from build123d import *

# Parameters (mm, degrees)
SKETCH1_W           = 200
SKETCH1_H           = 10
BOSS_EXTRUDE1_DEPTH = 66.54
CUT_EXTRUDE1_REACH  = 122.219
SKETCH2_R           = 1.5
LPATTERN1_COUNT     = 4
LPATTERN1_PITCH     = 64
SKETCH3_W           = 200
SKETCH3_H           = 10
CUT_EXTRUDE2_DEPTH  = 3
SKETCH4_W           = 3
SKETCH4_H           = 56.54
BOSS_EXTRUDE2_DEPTH = 8
CUT_EXTRUDE3_REACH  = 213.179
SKETCH5_R           = 1.5


with BuildPart() as part:
    # Sketch1 → Boss-Extrude1 (new body)
    with BuildSketch(Plane(origin=(0, 0, 0), x_dir=(1, 0, 0), z_dir=(0, 1, 0))):
        Rectangle(SKETCH1_W, SKETCH1_H)
    extrude(amount=BOSS_EXTRUDE1_DEPTH)

    # Sketch2 → Cut-Extrude1 (cut, up to next)
    with BuildSketch(Plane(origin=(0, 66.54, 0), x_dir=(1, 0, 0), z_dir=(0, 1, 0)), mode=Mode.PRIVATE) as cut_extrude1_sk1:
        with Locations(Location((-96, 0, 0), (0, 0, 270))):
            Circle(SKETCH2_R)
    cut_extrude1_tool1 = extrude(cut_extrude1_sk1.sketch, amount=-CUT_EXTRUDE1_REACH, mode=Mode.PRIVATE) & part.part
    cut_extrude1 = cut_extrude1_tool1.solids().sort_by_distance((-96, 66.54, 0))[0]
    add(cut_extrude1, mode=Mode.SUBTRACT)

    # LPattern1: Cut-Extrude1 ×4
    with Locations(*[(i * LPATTERN1_PITCH, 0, 0) for i in range(1, LPATTERN1_COUNT)]):
        add(cut_extrude1, mode=Mode.SUBTRACT)

    # Sketch3 → Cut-Extrude2 (cut)
    with BuildSketch(Plane.XY.offset(5)):
        with Locations((0, 5)):
            Rectangle(SKETCH3_W, SKETCH3_H)
    extrude(amount=-CUT_EXTRUDE2_DEPTH, mode=Mode.SUBTRACT)

    # Sketch4 → Boss-Extrude2 (add)
    with BuildSketch(Plane.XY.offset(5)):
        with Locations((-98.5, 38.27)):
            Rectangle(SKETCH4_W, SKETCH4_H)
    extrude(amount=BOSS_EXTRUDE2_DEPTH)

    # Sketch5 → Cut-Extrude3 (cut, up to next)
    with BuildSketch(Plane.ZY.offset(100), mode=Mode.PRIVATE) as cut_extrude3_sk1:
        with Locations((9, 58.27)):
            Circle(SKETCH5_R)
    cut_extrude3_tool1 = extrude(cut_extrude3_sk1.sketch, amount=-CUT_EXTRUDE3_REACH, mode=Mode.PRIVATE) & part.part
    # Sketch5 → Cut-Extrude3 (cut, up to next)
    with BuildSketch(Plane.ZY.offset(100), mode=Mode.PRIVATE) as cut_extrude3_sk2:
        with Locations((9, 13.27)):
            Circle(SKETCH5_R)
    cut_extrude3_tool2 = extrude(cut_extrude3_sk2.sketch, amount=-CUT_EXTRUDE3_REACH, mode=Mode.PRIVATE) & part.part
    add(cut_extrude3_tool1.solids().sort_by_distance((-100, 58.27, 9))[0], mode=Mode.SUBTRACT)
    add(cut_extrude3_tool2.solids().sort_by_distance((-100, 13.27, 9))[0], mode=Mode.SUBTRACT)


solid = part.part
Part model, mm, in its own coordinate system. A direction names the side the tool comes from. Round coordinates to 2 decimals unless told otherwise and drop trailing zeros. Write each loop counter-clockwise with the first axis right and the second up, starting at its lowest first coordinate (ties: lowest second). Pieces come first, ordered by that corner, then holes. Notation, with made-up numbers: M 22,75 L 28,75 A24 ccw 28,109 Z; hole C 27,11 d2. An arc over 180 degrees is marked long. Return JSON: item names as keys, results as strings. Group by question number.
(1) Drill centre lines: probe 1 along X at (y, z) = (43, 0); probe 2 along Z at (x, y) = (96, 28); probe 3 along X at (y, z) = (23.5, -0.5). Where is each one in solid material? Low to high.
(2) Saw through at A-A on x = 47. Write the cut outline in (y, z), then the cut area to 3 significant figures.
(3) Pin check, flat tips, straight feed: pin 1 Ø9 at (y, z) = (25, 10.5) entering from +X; pin 2 Ø6 at (x, y) = (-33.5, 38.5) entering from +Z; pin 3 Ø8 at (x, y) = (46, 5) entering from +Z; pin 4 Ø4 at (x, z) = (32, 0) entering from +Y. Stop position of each tip, or through.
(4) Which spindle directions (+Z, -Z, +X, -X, +Y, -Y) get a long thin tool onto all of the face, cutting with end or side? Do faces 1 (the face through (100, 33, 0)), 2 (the face through (-1, 5, 2)), 3 (the face through (-97, 38, 9)). Say none if no direction does.
Returned:
{
 "1": {"probe 1": "-100 to -97.5, -94.5 to -33.5, -30.5 to 30.5, 33.5 to 94.5, 97.5 to 100", "probe 2": "-5 to -1.5, 1.5 to 5", "probe 3": "-100 to -97.41, -94.59 to -33.41, -30.59 to 30.59, 33.41 to 94.59, 97.41 to 100"},
 "2": {"outline": "M 0,-5 L 66.54,-5 L 66.54,5 L 10,5 L 10,2 L 0,2 Z", "area": "635 mm²"},
 "3": {"pin 1": "x = -97", "pin 2": "z = 5", "pin 3": "z = 2", "pin 4": "y = 66.54"},
 "4": {"face 1": "+Z, -Z, +X, +Y, -Y", "face 2": "+Z, +X, -X, -Y", "face 3": "+Z, +X, +Y, -Y"}
}
